```python
from build123d import *

# Parameters (mm, degrees)
SKETCH1_W           = 19.05
SKETCH1_H           = 19.05
SKETCH1_W_2         = 15.875
SKETCH1_H_2         = 15.875
BOSS_EXTRUDE1_DEPTH = 495.3
SKETCH2_R           = 3.96875
CUT_EXTRUDE1_DEPTH  = 1.5875
CUT_EXTRUDE2_REACH  = 21.05
SKETCH3_R           = 0.889


with BuildPart() as part:
    # Sketch1 → Boss-Extrude1 (new body)
    with BuildSketch(Plane(origin=(0, 0, 0), x_dir=(1, 0, 0), z_dir=(0, 1, 0))):
        Rectangle(SKETCH1_W, SKETCH1_H)
        Rectangle(SKETCH1_W_2, SKETCH1_H_2, mode=Mode.SUBTRACT)
    extrude(amount=BOSS_EXTRUDE1_DEPTH)

    # Sketch2 → Cut-Extrude1 (cut)
    with BuildSketch(Plane.XY.offset(9.525)):
        with Locations((-1.095375, 11.4523012)):
            Circle(SKETCH2_R)
    extrude(amount=-CUT_EXTRUDE1_DEPTH, mode=Mode.SUBTRACT)

    # Sketch3 → Cut-Extrude2 (cut, up to next)
    with BuildSketch(Plane.ZY.offset(9.525), mode=Mode.PRIVATE) as cut_extrude2_sk1:
        with Locations((0, 9.525)):
            Circle(SKETCH3_R)
    cut_extrude2_tool1 = extrude(cut_extrude2_sk1.sketch, amount=-CUT_EXTRUDE2_REACH, mode=Mode.PRIVATE) & part.part
    add(cut_extrude2_tool1.solids().sort_by_distance((-9.525, 9.525, 0))[0], mode=Mode.SUBTRACT)


solid = part.part
```
Can you work these out from the model? Positions are in its coordinate system, mm. A direction names the side the tool comes from. Round coordinates to 2 decimals unless told otherwise and drop trailing zeros. Loops run counter-clockwise (first coordinate to the right, second up) from the corner with the lowest first, then second, coordinate; pieces in that order, holes last.
Item 1: Will these pins go through, and if not, where does the flat tip stop? pin 1 Ø3 at (x, z) = (0.5, -6) entering from -Y; pin 2 Ø10 at (x, z) = (-4, -1.5) entering from -Y.
Item 2: Which directions (+Z, -Z, +X, -X, +Y, -Y) give clear straight access to the entire face, cutting with the end or side of a thin tool? Please do faces 5 (the cylindrical face through (-1.96, 7.58, 8.74)), 6 (the flat face through (7.938, 244, 0)), 7 (the flat face through (-9, 495.3, 0)).
Item 3: Please list where these lines run through material, in increasing order: L1, parallel to X at y = 219, z = 2.25 (1 decimal); L2, parallel to Y at x = -9.1, z = 0.
Item 4: If we mould it in two halves opening along Z, with no side actions, what happens to faces 1 (the flat face through (-7.938, 244, 0)), 2 (the flat face through (-9.525, 244, 0)), 3 (the flat face through (0, 244, -9.525)), 4 (the flat face through (0, 244, 7.938))? For each: +Z half, -Z half, draft (parallel to the pull), parting line (faces both ways), or undercut.
Item 5: Suppose I cut it at A-A, the plane z = 4.5. Write out the boundary of the cut face in (x, y) (1 decimal), then the cut area to 3 significant figures.
Item 6: Suppose I cut it at B-B, the plane y = 219. Write out the boundary of the cut face in (x, z) (1 decimal).
Reported:
1. pin 1: passes through
1. pin 2: stops at y = 0
2. face 5: +Z
2. face 6: +Y, -Y
2. face 7: +Z, -Z, +X, -X, +Y
3. L1: x = -9.5 to -7.9, 7.9 to 9.5
3. L2: y = 0 to 8.64, 10.41 to 495.3
4. face 1: undercut
4. face 2: draft
4. face 3: -Z half
4. face 4: undercut
5. outline: (-9.5, 0) - (-7.9, 0) - (-7.9, 495.3) - (-9.5, 495.3) - close; (7.9, 0) - (9.5, 0) - (9.5, 495.3) - (7.9, 495.3) - close
5. area: 1,570 mm2
6. outline: (-9.5, -9.5) - (9.5, -9.5) - (9.5, 9.5) - (-9.5, 9.5) - close; hole (-7.9, -7.9) - (7.9, -7.9) - (7.9, 7.9) - (-7.9, 7.9) - close
